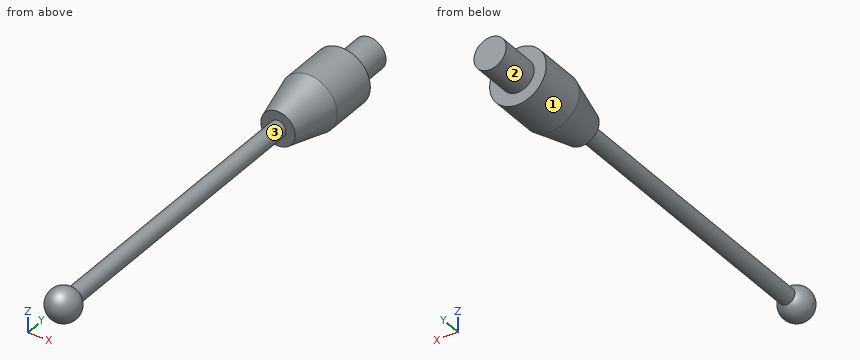
```python
from build123d import *

# Parameters (mm, degrees)
SKETCH3_R           = 2
BOSS_EXTRUDE1_DEPTH = 5


with BuildPart() as part:
    # Sketch2 → Revolve1 (revolve)
    with BuildSketch(Plane.XY, mode=Mode.PRIVATE) as revolve1_sk:
        with BuildLine():
            Line((1, 1.732050808), (1, 38.5))
            Line((1, 38.5), (2.123066207, 38.5))
            Line((2.123066207, 38.5), (3.5, 44.068591296))
            Line((3.5, 44.068591296), (3.5, 50))
            Line((3.5, 50), (0, 50))
            Line((0, 50), (0, -2))
            ThreePointArc((0, -2), (1.931851653, -0.51763809), (1, 1.732050808))
        make_face()
    revolve(revolve1_sk.sketch.rotate(Axis((0, -2, 0), (0, 1, 0)), 90), axis=Axis((0, -2, 0), (0, 1, 0)))

    # Sketch3 → Boss-Extrude1 (add)
    with BuildSketch(Plane(origin=(0, 50, 0), x_dir=(1, 0, 0), z_dir=(0, 1, 0))):
        with Locations(Location((0, 0, 0), (0, 0, 90))):
            Circle(SKETCH3_R)
    extrude(amount=BOSS_EXTRUDE1_DEPTH)


solid = part.part
```
Part model, mm, in its own coordinate system. Face numbers are marked on the shaded views. A direction names the side the tool comes from. Round coordinates to 2 decimals unless told otherwise and drop trailing zeros. Order: outer loops, then holes, each group sorted by start corner. A loop starts at its lowest first (then second) coordinate and runs counter-clockwise, first axis right, second up. Notation, with made-up numbers: M -12.5,76.25 L 6.5,76.25 A22 ccw 6.5,107.25 Z; hole C 37.5,-16 d1. An arc over 180 degrees is marked long. Answer in a Markdown table with one row per item. Add a question column.
Q1. Wall check: L1, parallel to Y at x = 1.25, z = -1; L2, parallel to Z at x = 0.5, y = 25; L3, parallel to Y at x = 0.75, z = -1. Give the ranges that are in metal, low to high. Write a range as from..to.
Q2. Cut at A-A on z = 0. Give the cut face in (x, y), and give its area (3 significant figures).
Q3. 3-axis set-ups, long thin cutter, end or side, ignore diameter. For the marked faces 1, 2 and 3: which of +Z, -Z, +X, -X, +Y, -Y reach the whole face in a straight line?
Q4. Cut at C-C on y = 47. Give the cut face in (x, z).
Q5. Cut at B-B on x = 0. Give the cut face in (y, z), and give its area (3 significant figures).
Q6. Pin check, flat tips, straight feed: pin 1 (3 mm diameter, centred on x = 1.5, y = 39, fed in from +Z); pin 2 (3 mm diameter, centred on x = -2, y = 7, fed in from +Z); pin 3 (3 mm diameter, centred on x = 1.5, y = 11, fed in from +Z). Stop position of each tip, or through.
Q7. Cut at D-D on y = 7.5. Give the cut face in (x, z).
Established:
| question | item | result |
|---|---|---|
| 1 | L1 | y = -1.2..1.2, 38.5..55 |
| 1 | L2 | z = -0.87..0.87 |
| 1 | L3 | y = -1.56..1.56, 38.5..55 |
| 2 | outline | M -3.5,44.07 L -2.12,38.5 L -1,38.5 L -1,1.73 A2 ccw long 1,1.73 L 1,38.5 L 2.12,38.5 L 3.5,44.07 L 3.5,50 L 2,50 L 2,55 L -2,55 L -2,50 L -3.5,50 Z |
| 2 | area | 179 mm2 |
| 3 | face 1 | +Y, -Y |
| 3 | face 2 | +Y |
| 3 | face 3 | none |
| 4 | outline | C 0,0 d7 |
| 5 | outline | M 1.73,-1 L 38.5,-1 L 38.5,-2.12 L 44.07,-3.5 L 50,-3.5 L 50,-2 L 55,-2 L 55,2 L 50,2 L 50,3.5 L 44.07,3.5 L 38.5,2.12 L 38.5,1 L 1.73,1 A2 ccw long Z |
| 5 | area | 179 mm2 |
| 6 | pin 1 | stops at z = 2.47 |
| 6 | pin 2 | stops at z = 0.87 |
| 6 | pin 3 | stops at z = 1 |
| 7 | outline | C 0,0 d2 |
